from build123d import *

# Parameters (mm, degrees)
F0_R     = 1.25
F1_DEPTH = 6
F2_R     = 0.75
F3_DEPTH = 12
F4_SIZE2 = 0.3
F4_SIZE  = 1


with BuildPart() as f1:
    # F0 (on Top) → F1 (new body, symmetric)
    with BuildSketch(Plane.XY):
        Circle(F0_R)
    extrude(amount=F1_DEPTH, both=True)

    # F2 (on face) → F3 (cut, through all)
    with BuildSketch(Plane(origin=(0, 0, -6), x_dir=(1, 0, 0), z_dir=(0, 0, -1))):
        Circle(F2_R)
    extrude(amount=-F3_DEPTH, mode=Mode.SUBTRACT)

    # F4
    f4_edges = [f1.edges().sort_by_distance(p)[0] for p in [
        (-1.25, 0, -6),
        (-1.25, 0, 6),
    ]]
    chamfer(f4_edges, length=F4_SIZE, length2=F4_SIZE2)


solid = f1.part
Model file for the job. Use its own axes, mm. Give positions to 0.01 mm unless a question says otherwise; leave off trailing zeros. Loops run counter-clockwise (first coordinate to the right, second up) from the corner with the lowest first, then second, coordinate; pieces in that order, holes last. Notation, with made-up numbers: (2.25, 19) -> (46.25, 19) arc R25 cw to (46.25, 44) -> close; hole circle Ø1 at (16.25, 88). An arc over 180 degrees is marked (long way). Use a Markdown table: item, result. Add a question column.
(1) Slice it at A-A on y = 0. List the corners of the cut face in (x, z), and give its area (3 significant figures).
(2) Drop a flat-ended pin along its axis: pin 1 Ø1.5 at (x, y) = (0.5, 0.5) entering from -Z. Give the stop position or say it passes through.
(3) Mould opens along X. For faces 1 (the cylindrical face through (-0.75, -0.03, -0.08)), 2 (the cylindrical face through (-0.27, -1.22, 0.07)) say: +X half, -X half, draft (parallel to the pull), parting line (faces both ways), or undercut.
(4) Slice it at C-C on z = 4.5. List the corners of the cut face in (x, y), and give its area (3 significant figures).
(5) Wall check: line 1 along Y through (x, z) = (0, -1.25); line 2 along Y through (x, z) = (0.5, 1.25); line 3 along X through (y, z) = (0.1, 5). Give the ranges that are in metal, low to high.
Filled sheet:
| question | item | result |
|---|---|---|
| 1 | outline | (-1.25, -5) -> (-0.95, -6) -> (-0.75, -6) -> (-0.75, 6) -> (-0.95, 6) -> (-1.25, 5) -> close; (0.75, -6) -> (0.95, -6) -> (1.25, -5) -> (1.25, 5) -> (0.95, 6) -> (0.75, 6) -> close |
| 1 | area | 11.4 mm2 |
| 2 | pin 1 | z = -6 |
| 3 | face 1 | undercut |
| 3 | face 2 | parting line |
| 4 | outline | circle Ø2.5 at (0, 0); hole circle Ø1.5 at (0, 0) |
| 4 | area | 3.14 mm2 |
| 5 | line 1 | -1.25 to -0.75, 0.75 to 1.25 |
| 5 | line 2 | -1.15 to -0.56, 0.56 to 1.15 |
| 5 | line 3 | -1.25 to -0.74, 0.74 to 1.25 |
